Geometry check sheet. Reference: the model listing, model coordinates, mm. Face numbers are marked on the shaded views. A direction names the side the tool comes from. Give positions to 0.01 mm unless a question says otherwise; leave off trailing zeros.
(1) Mould release check, pull along X, two halves, no side actions. Record for the marked faces 1 and 2: +X half, -X half, draft (parallel to the pull), parting line (faces both ways), or undercut.
(2) Thickness scan on line 1 along X through (y, z) = (-3.75, 0.7); line 2 along X through (y, z) = (1, 1.2); line 3 along X through (y, z) = (-5, 1.95). Record the ranges inside material, lowest first.
(3) Tool access check on the marked faces 3 and 4. Record the directions out of +Z, -Z, +X, -X, +Y, -Y that give a thin tool (end or side, any length) a straight path to the whole face; none if there is none.
(4) Depth check by flat-ended pin: P1, Ø1, axis at y = 4, z = 1, coming from the +X side; P2, Ø0.7, axis at x = -1.5, z = 1.5, coming from the -Y side. Enter the tip coordinate at first touch or a pass-through.
(5) Cross-section at A-A (y = 0). Count the separate pieces of the cut face and the enclosed holes in it, and give its area (3 significant figures).
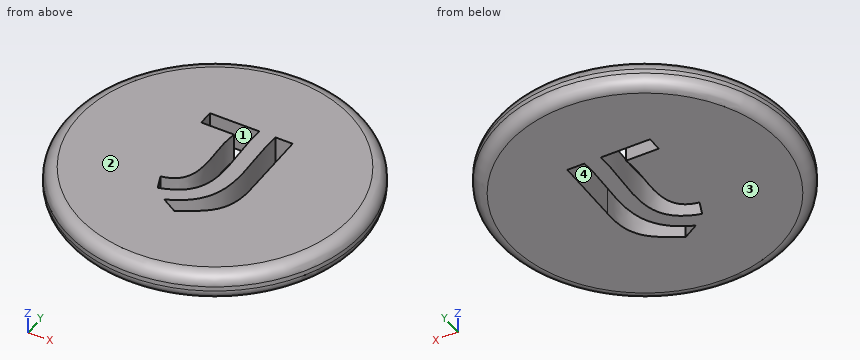
```python
from build123d import *

# Parameters (mm, degrees)
F0_R     = 12.125
F1_DEPTH = 2.38
F2_R     = 1


with BuildPart() as f1:
    # F0 (on Top) → F1 (new body)
    with BuildSketch(Plane.XY):
        Circle(F0_R)
        with BuildLine():
            add(Edge.make_bspline(
                [(2.036581, 4.983431), (1.639226, 1.080341), (3.435804, -3.024245), (-1.276224, -4.923354)],
                knots=[0, 0, 0, 0, 10.446007, 10.446007, 10.446007, 10.446007], degree=3))
            Line((2.036581, 4.983431), (3.429502, 4.983431))
            Line((3.429502, 4.983431), (3.429502, -0.670792))
            add(Edge.make_bspline(
                [(3.429502, -0.670792), (3.556498, -4.298475), (1.374324, -4.697141), (0, -5.683316)],
                knots=[0, 0, 0, 0, 6.073458, 6.073458, 6.073458, 6.073458], degree=3))
            Line((0, -5.683316), (-1.276224, -4.923354))
        make_face(mode=Mode.SUBTRACT)
        with BuildLine():
            Line((-3.320744, 3.784657), (-3.320744, 4.989943))
            Line((-3.320744, 4.989943), (0.701266, 4.989943))
            add(Edge.make_bspline(
                [(0.701266, 4.989943), (0.401681, 1.040562), (2.123402, -2.876976), (-2.325447, -4.02479)],
                knots=[0, 0, 0, 0, 9.509279, 9.509279, 9.509279, 9.509279], degree=3))
            Line((-2.325447, -4.02479), (-2.794653, -2.832613))
            add(Edge.make_bspline(
                [(-0.644522, 3.784657), (-1.176108, 1.48316), (0.391602, -2.325576), (-2.794653, -2.832613)],
                knots=[0, 0, 0, 0, 6.957825, 6.957825, 6.957825, 6.957825], degree=3))
            Line((-0.644522, 3.784657), (-3.320744, 3.784657))
        make_face(mode=Mode.SUBTRACT)
    extrude(amount=F1_DEPTH)

    # F2
    f2_edges = [f1.edges().sort_by_distance(p)[0] for p in [
        (-12.125, 0, 2.38),
        (-12.125, 0, 0),
    ]]
    fillet(f2_edges, radius=F2_R)


solid = f1.part
```
Reply:
1. face 1: undercut
1. face 2: draft
2. line 1: x = -11.48 to -2.43, -1.49 to 0.63, 2.65 to 11.48
2. line 2: x = -12.08 to -0.72, 0.78 to 2.05, 3.43 to 12.08
2. line 3: x = -10.85 to -1.15, 1.12 to 10.85
3. face 3: -Z, +X, -X, +Y, -Y
3. face 4: +Z, -Z
4. P1: stops at x = 11.61
4. P2: stops at y = -12.07
5. separate pieces: 3
5. enclosed holes: 0
5. area: 50.0 mm2
